Verification items for the finished model (mm, model axes). Give positions to 0.01 mm unless a question says otherwise; leave off trailing zeros. Write each loop counter-clockwise with the first axis right and the second up, starting at its lowest first coordinate (ties: lowest second). Pieces come first, ordered by that corner, then holes.
Autodesk Inventor part; units mm, degrees
ref_plane "YZ Plane" through (0, 0, 0) normal (1, 0, 0) x (0, 1, 0)
ref_plane "XZ Plane" through (0, 0, 0) normal (0, 1, 0) x (-1, 0, 0)
ref_plane "XY Plane" through (0, 0, 0) normal (0, 0, 1) x (1, 0, 0)
sketch "Sketch1" plane through (0, 0, 0) normal (0, 0, 1) x (1, 0, 0)
  line L0 (-31.4222, 23.2631) -> (19.3778, 23.2631)
  line L1 (19.3778, 23.2631) -> (19.3778, -21.1869)
  line L2 (19.3778, -21.1869) -> (-31.4222, -21.1869)
  line L3 (-31.4222, -21.1869) -> (-31.4222, 23.2631)
  point P0 (0, 0)
  dimension "d0" = 44.45
  dimension "d1" = 50.8
extrude "Extrusion1" add sketch "Sketch1" along normal blind 6.35
sketch "Sketch2" plane through (0, 0, 6.35) normal (0, 0, 1) x (1, 0, 0)
  line L0 (-31.4222, -21.1869) -> (19.3778, -21.1869)
  line L1 (19.3778, -21.1869) -> (19.3778, -27.5369)
  line L2 (19.3778, -27.5369) -> (-31.4222, -27.5369)
  line L3 (-31.4222, -27.5369) -> (-31.4222, -21.1869)
  line L4 (19.3778, -21.1869) -> (19.3778, 23.2631)
  line L5 (-31.4222, 23.2631) -> (-31.4222, -21.1869)
  line L6 (-31.4222, -21.1869) -> (19.3778, -21.1869)
  point P0 (0, 0)
  dimension "d4" = 0
  dimension "d5" = 0
  dimension "d6" = 6.35
  dimension "d7" = 0
extrude "Extrusion2" add sketch "Sketch2" against normal blind 57.15
sketch "Sketch3" plane through (0, 0, 6.35) normal (0, 0, 1) x (1, 0, 0)
  line L0 (19.3778, 23.2631) -> (-31.4222, 23.2631)
  line L1 (-31.4222, 23.2631) -> (-31.4222, -27.5369)
  line L2 (19.3778, 23.2631) -> (19.3778, -27.5369)
  point P0 (0, 0)
  point P1 (-21.2622, 19.4531)
  point P2 (-21.2622, -8.4869)
  point P3 (7.9478, 19.4531)
  point P4 (7.9478, -8.4869)
  dimension "d10" = 29.21
  dimension "d11" = 0
  dimension "d12" = 0
  dimension "d13" = 0
  dimension "d14" = 27.94
  dimension "d15" = 3.81
  dimension "d16" = 10.16
  dimension "d17" = 11.43
  dimension "d25" = 0
hole "Hole1" at (-21.2622, 19.4531, 6.35) at (-21.2622, -8.4869, 6.35) at (7.9478, 19.4531, 6.35) at (7.9478, -8.4869, 6.35) direction (0, 0, -1) diameter 3.81 depth 25.4 tip angle 118
sketch "Sketch4" plane through (0, 0, 6.35) normal (0, 0, 1) x (1, 0, 0)
  circle A0 centre (-21.2622, 19.4531) radius 1.905
  point P0 (0, 0)
  point P1 (-18.7222, 15.6431)
  point P2 (9.2178, 15.6431)
  point P3 (9.2178, -13.5669)
  point P4 (-18.7222, -13.5669)
  dimension "d26" = 0
  dimension "d27" = 0
  dimension "d28" = 0
  dimension "d29" = 0
  dimension "d30" = 29.21
  dimension "d31" = 27.94
  dimension "d42" = 2.54
  dimension "d43" = 3.81
hole "Hole2" at (-18.7222, 15.6431, 6.35) at (9.2178, 15.6431, 6.35) at (9.2178, -13.5669, 6.35) at (-18.7222, -13.5669, 6.35) direction (0, 0, -1) diameter 3.81 depth 25.4 tip angle 118
sketch "Sketch5" plane through (-31.4222, -21.1869, 0) normal (0, 1, 0) x (1, 0, 0)
  line L0 (50.8, 0) -> (50.8, 50.8)
  line L1 (0, 50.8) -> (50.8, 50.8)
  point P0 (31.4222, 0)
  point P1 (44.45, 44.45)
  point P2 (44.45, 36.83)
  point P3 (44.45, 29.21)
  point P4 (44.45, 21.59)
  point P5 (44.45, 13.97)
  point P6 (44.45, 6.35)
  point P7 (36.83, 6.35)
  point P8 (36.83, 13.97)
  point P9 (36.83, 21.59)
  point P10 (36.83, 29.21)
  point P11 (36.83, 36.83)
  point P12 (36.83, 44.45)
  point P13 (29.21, 6.35)
  point P14 (29.21, 13.97)
  point P15 (29.21, 21.59)
  point P16 (29.21, 29.21)
  point P17 (29.21, 36.83)
  point P18 (29.21, 44.45)
  point P19 (21.59, 6.35)
  point P20 (21.59, 13.97)
  point P21 (21.59, 21.59)
  point P22 (21.59, 29.21)
  point P23 (21.59, 36.83)
  point P24 (21.59, 44.45)
  point P25 (13.97, 6.35)
  point P26 (13.97, 13.97)
  point P27 (13.97, 21.59)
  point P28 (13.97, 29.21)
  point P29 (13.97, 36.83)
  point P30 (13.97, 44.45)
  point P31 (6.35, 6.35)
  point P32 (6.35, 13.97)
  point P33 (6.35, 21.59)
  point P34 (6.35, 29.21)
  point P35 (6.35, 36.83)
  point P36 (6.35, 44.45)
  dimension "d44" = 6.35
  dimension "d45" = 6.35
  dimension "d48" = 7.62
  dimension "d58" = 7.62
hole "Hole3" at (13.0278, -21.1869, -44.45) at (13.0278, -21.1869, -36.83) at (13.0278, -21.1869, -29.21) at (13.0278, -21.1869, -21.59) at (13.0278, -21.1869, -13.97) at (13.0278, -21.1869, -6.35) at (5.4078, -21.1869, -6.35) at (5.4078, -21.1869, -13.97) at (5.4078, -21.1869, -21.59) at (5.4078, -21.1869, -29.21) at (5.4078, -21.1869, -36.83) at (5.4078, -21.1869, -44.45) at (-2.2122, -21.1869, -6.35) at (-2.2122, -21.1869, -13.97) at (-2.2122, -21.1869, -21.59) at (-2.2122, -21.1869, -29.21) at (-2.2122, -21.1869, -36.83) at (-2.2122, -21.1869, -44.45) at (-9.8322, -21.1869, -6.35) at (-9.8322, -21.1869, -13.97) at (-9.8322, -21.1869, -21.59) at (-9.8322, -21.1869, -29.21) at (-9.8322, -21.1869, -36.83) at (-9.8322, -21.1869, -44.45) at (-17.4522, -21.1869, -6.35) at (-17.4522, -21.1869, -13.97) at (-17.4522, -21.1869, -21.59) at (-17.4522, -21.1869, -29.21) at (-17.4522, -21.1869, -36.83) at (-17.4522, -21.1869, -44.45) at (-25.0722, -21.1869, -6.35) at (-25.0722, -21.1869, -13.97) at (-25.0722, -21.1869, -21.59) at (-25.0722, -21.1869, -29.21) at (-25.0722, -21.1869, -36.83) at (-25.0722, -21.1869, -44.45) direction (0, -1, 0) diameter 3.81 depth 25.4 tip angle 118
properties part number "LidarMount2"
Item 1: Depth check by flat-ended pin: pin 1 (4 mm diameter, centred on x = 0.5, y = 6, fed in from -Z); pin 2 (3.5 mm diameter, centred on x = -25.07, z = -44.45, fed in from +Y); pin 3 (8 mm diameter, centred on x = -6, z = -42.5, fed in from +Y). Enter the tip coordinate at first touch or a pass-through.
Answer key:
pin 1: stops at z = 0
pin 2: passes through
pin 3: stops at y = -21.19
Item 2: Release check for a two-part mould opening along Y. For faces 1 (the face through (-15.59, -24.41, -22)), 2 (the face through (-6, 23.263, 3)), 3 (the face through (-20.61, 15.89, 3.13)) record: released by +Y, released by -Y, zero draft, split by the parting line, or undercut.
Answer key:
face 1: zero draft
face 2: released by +Y
face 3: undercut
Item 3: Sectioned sample at D-D on y = 9. Record the cut outline in (x, z).
Answer key:
outline: (-31.42, 0) - (19.38, 0) - (19.38, 6.35) - (-31.42, 6.35) - close
Item 4: Sectioned sample at A-A on z = -6.35. Record the cut outline in (x, y), then the cut area to 3 significant figures.
Answer key:
outline: (-31.42, -27.54) - (-26.98, -27.54) - (-26.98, -21.19) - (-31.42, -21.19) - close; (-23.17, -27.54) - (-19.36, -27.54) - (-19.36, -21.19) - (-23.17, -21.19) - close; (-15.55, -27.54) - (-11.74, -27.54) - (-11.74, -21.19) - (-15.55, -21.19) - close; (-7.93, -27.54) - (-4.12, -27.54) - (-4.12, -21.19) - (-7.93, -21.19) - close; (-0.31, -27.54) - (3.5, -27.54) - (3.5, -21.19) - (-0.31, -21.19) - close; (7.31, -27.54) - (11.12, -27.54) - (11.12, -21.19) - (7.31, -21.19) - close; (14.93, -27.54) - (19.38, -27.54) - (19.38, -21.19) - (14.93, -21.19) - close
area: 177 mm2
Item 5: Scan lines: line 1 along X through (y, z) = (15.5, 2); line 2 along Z through (x, y) = (16, -11.5); line 3 along Y through (x, z) = (-10, -3.5). Record each from-to range of solid material in increasing order.
Answer key:
line 1: x = -31.42 to -20.62, -16.82 to 7.32, 11.12 to 19.38
line 2: z = 0 to 6.35
line 3: y = -27.54 to -21.19
Item 6: Sectioned sample at B-B on z = 2. State how many separate pieces and enclosed holes the cut face has, then the cut area to 3 significant figures.
Answer key:
separate pieces: 1
enclosed holes: 8
area: 2,490 mm2
Item 7: Sectioned sample at C-C on x = -14. Record the cut outline in (y, z).
Answer key:
outline: (-27.54, -50.8) - (-21.19, -50.8) - (-21.19, 0) - (23.26, 0) - (23.26, 6.35) - (-27.54, 6.35) - close
